from build123d import *

# Parameters (mm, degrees)
BOSS_EXTRUDE1_DEPTH  = 100
BOSS_EXTRUDE2_DEPTH  = 10
BOSS_EXTRUDE2_DRAFT  = 45
SKETCH3_R            = 34.5
BOSS_EXTRUDE3_DEPTH  = 10
SKETCH4_R            = 31
BOSS_EXTRUDE4_DEPTH  = 30
SKETCH5_R            = 2.5
SKETCH5_R_2          = 2
BOSS_EXTRUDE5_DEPTH  = 1
CIRPATTERN1_COUNT    = 12
BOSS_EXTRUDE6_DEPTH  = 100
SKETCH7_R            = 31
BOSS_EXTRUDE7_DEPTH  = 10
SKETCH8_R            = 30
BOSS_EXTRUDE8_DEPTH  = 1
SKETCH9_R            = 31
BOSS_EXTRUDE9_DEPTH  = 10
SKETCH11_R           = 42.5
BOSS_EXTRUDE10_DEPTH = 10.5
BOSS_EXTRUDE11_DEPTH = 35
BOSS_EXTRUDE12_DEPTH = 40
CUT_EXTRUDE1_DEPTH   = 40
SKETCH16_R           = 15
CUT_EXTRUDE2_DEPTH   = 20
SKETCH17_R           = 15
CUT_EXTRUDE3_DEPTH   = 20


with BuildPart() as part:
    # Sketch1 → Boss-Extrude1 (new body)
    with BuildSketch(Plane(origin=(0, 0, 0), x_dir=(1, 0, 0), z_dir=(0, 1, 0))):
        with BuildLine():
            Line((-37.5, 45), (37.5, 45))
            ThreePointArc((37.5, 45), (45.880962103, 0), (37.5, -45))
            Line((37.5, -45), (-37.5, -45))
            ThreePointArc((-37.5, -45), (-45.880962103, 0), (-37.5, 45))
        make_face()
    extrude(amount=BOSS_EXTRUDE1_DEPTH)


with BuildPart() as boss_extrude2_tool:
    # Sketch2 → Boss-Extrude2 (with draft: the straight prism first)
    with BuildSketch(Plane(origin=(0, 100, 0), x_dir=(1, 0, 0), z_dir=(0, 1, 0))):
        with BuildLine():
            Line((37.5, 45), (-37.5, 45))
            ThreePointArc((-37.5, 45), (-45.880962103, 0), (-37.5, -45))
            Line((-37.5, -45), (37.5, -45))
            ThreePointArc((37.5, -45), (45.880962103, 0), (37.5, 45))
        make_face()
    extrude(amount=BOSS_EXTRUDE2_DEPTH)
    # Boss-Extrude2: the draft: its side faces are tilted about the plane it starts from
    boss_extrude2_sides = [boss_extrude2_tool.faces().sort_by_distance(p)[0] for p in [
        (0, 105, -45),
        (-45.880962103, 105, 0),
        (0, 105, 45),
        (45.880962103, 105, 0),
    ]]
    draft(boss_extrude2_sides, Plane(origin=(0, 100, 0), x_dir=(1, 0, 0), z_dir=(0, 1, 0)), BOSS_EXTRUDE2_DRAFT)


with BuildPart() as part_1:
    add(part.part)

    # Boss-Extrude2: add boss_extrude2_tool
    add(boss_extrude2_tool.part)

    # Sketch3 → Boss-Extrude3 (add)
    with BuildSketch(Plane(origin=(0, 110, 0), x_dir=(1, 0, 0), z_dir=(0, 1, 0))):
        with Locations(Location((0, 0, 0), (0, 0, 270))):
            Circle(SKETCH3_R)
    extrude(amount=BOSS_EXTRUDE3_DEPTH)

    # Sketch4 → Boss-Extrude4 (add)
    with BuildSketch(Plane(origin=(0, 120, 0), x_dir=(1, 0, 0), z_dir=(0, 1, 0))):
        with Locations(Location((0, 0, 0), (0, 0, 270))):
            Circle(SKETCH4_R)
    extrude(amount=BOSS_EXTRUDE4_DEPTH)

    # Sketch5 → Boss-Extrude5 (add)
    with BuildSketch(Plane(origin=(0, 150, 0), x_dir=(1, 0, 0), z_dir=(0, 1, 0))):
        with Locations(Location((27, 0, 0), (0, 0, 270))):
            Circle(SKETCH5_R)
        with Locations(Location((27, 0, 0), (0, 0, 270))):
            Circle(SKETCH5_R_2, mode=Mode.SUBTRACT)
    boss_extrude5 = extrude(amount=BOSS_EXTRUDE5_DEPTH)

    # CirPattern1: Boss-Extrude5 ×12 about axis
    cirpattern1_axis = Axis((0, 0, 0), (0, 1, 0))
    for i in range(1, CIRPATTERN1_COUNT):
        add(boss_extrude5.rotate(cirpattern1_axis, i * 360 / CIRPATTERN1_COUNT))

    # Sketch6 → Boss-Extrude6 (add)
    with BuildSketch(Plane(origin=(0, 150, 0), x_dir=(1, 0, 0), z_dir=(0, 1, 0))):
        with BuildLine():
            Line((16, 17), (16, -17))
            ThreePointArc((16, -17), (0, -23.900331129), (-16, -17))
            Line((-16, -17), (-16, 17))
            ThreePointArc((-16, 17), (0, 23.900331129), (16, 17))
        make_face()
    extrude(amount=BOSS_EXTRUDE6_DEPTH)

    # Sketch7 → Boss-Extrude7 (add)
    with BuildSketch(Plane(origin=(0, 250, 0), x_dir=(1, 0, 0), z_dir=(0, 1, 0))):
        with Locations(Location((0, 0, 0), (0, 0, 270))):
            Circle(SKETCH7_R)
    extrude(amount=BOSS_EXTRUDE7_DEPTH)

    # Sketch8 → Boss-Extrude8 (add)
    with BuildSketch(Plane(origin=(0, 260, 0), x_dir=(1, 0, 0), z_dir=(0, 1, 0))):
        with Locations(Location((0, 0, 0), (0, 0, 270))):
            Circle(SKETCH8_R)
    extrude(amount=BOSS_EXTRUDE8_DEPTH)

    # Sketch9 → Boss-Extrude9 (add)
    with BuildSketch(Plane(origin=(0, 261, 0), x_dir=(1, 0, 0), z_dir=(0, 1, 0))):
        with Locations(Location((0, 0, 0), (0, 0, 270))):
            Circle(SKETCH9_R)
    extrude(amount=BOSS_EXTRUDE9_DEPTH)

    # Sketch11 → Boss-Extrude10 (add, symmetric)
    with BuildSketch(Plane.ZY.offset(-37.5)):
        Circle(SKETCH11_R)
    extrude(amount=BOSS_EXTRUDE10_DEPTH, both=True)

    # Sketch12 → Boss-Extrude11 (add)
    with BuildSketch(Plane.ZY.offset(-27)):
        with BuildLine():
            Line((-20, 0), (20, 0))
            Line((20, 0), (20, -30))
            ThreePointArc((20, -30), (0, -37.639320225), (-20, -30))
            Line((-20, -30), (-20, 0))
        make_face()
    extrude(amount=BOSS_EXTRUDE11_DEPTH)

    # Sketch14 → Boss-Extrude12 (add)
    with BuildSketch(Plane(origin=(0, 0, -20), x_dir=(-1, 0, 0), z_dir=(0, 0, -1))):
        with BuildLine():
            Line((8, 0), (8, -42))
            ThreePointArc((8, -42), (25.421855105, -23.929675658), (33, 0))
            Line((33, 0), (8, 0))
        make_face()
    extrude(amount=-BOSS_EXTRUDE12_DEPTH)

    # Sketch15 → Cut-Extrude1 (cut)
    with BuildSketch(Plane(origin=(-8, 0, 0), x_dir=(0, 0, -1), z_dir=(1, 0, 0))):
        with BuildLine():
            Line((-20, -30), (-20, -42))
            Line((-20, -42), (20, -42))
            Line((20, -42), (20, -30))
            ThreePointArc((20, -30), (0, -37.639320225), (-20, -30))
        make_face()
    extrude(amount=-CUT_EXTRUDE1_DEPTH, mode=Mode.SUBTRACT)

    # Sketch16 → Cut-Extrude2 (cut)
    with BuildSketch(Plane(origin=(0, 271, 0), x_dir=(1, 0, 0), z_dir=(0, 1, 0))):
        with Locations(Location((0, 0, 0), (0, 0, 270))):
            Circle(SKETCH16_R)
    extrude(amount=-CUT_EXTRUDE2_DEPTH, mode=Mode.SUBTRACT)

    # Sketch17 → Cut-Extrude3 (cut)
    with BuildSketch(Plane(origin=(48, 0, 0), x_dir=(0, 0, -1), z_dir=(1, 0, 0))):
        Circle(SKETCH17_R)
    extrude(amount=-CUT_EXTRUDE3_DEPTH, mode=Mode.SUBTRACT)


solid = part_1.part
For this review, take the finished solid that the model builds, in its own axes (mm). A direction names the side the tool comes from. Give positions to 0.01 mm unless a question says otherwise; leave off trailing zeros. Loops run counter-clockwise (first coordinate to the right, second up) from the corner with the lowest first, then second, coordinate; pieces in that order, holes last. Notation, with made-up numbers: M -33,24 L 23,24 A24 cw 23,58 Z; hole C -23,50.25 d8. An arc over 180 degrees is marked long. Answer as a JSON object with one key per item and string values. Group by question number.
Q1. Add section C-C on y = 67. Give the boundary of the cut face in (x, z).
Q2. Insertion check: P1, Ø2.5, axis at x = 27, z = 0, coming from the -Y side; P2, Ø9, axis at x = -5.5, y = -19, coming from the -Z side; P3, Ø1, axis at y = 67, z = 31, coming from the +X side. Each pin has a flat end and moves straight along its axis. Give the tip position at first contact, or say it passes through.
Q3. Add section B-B on y = 207.5. Give the boundary of the cut face in (x, z), and give its area (3 significant figures).
Q4. Tool access review of faces 4 (the cylindrical face through (39.69, -41.49, -9.21)), 5 (the flat face through (-32.1, 110, -13.1)), 6 (the flat face through (28, 260, -12)): name each direction out of +Z, -Z, +X, -X, +Y, -Y from which nothing blocks a thin tool from reaching the whole face with its end or side.
Q5. Add section D-D on y = -12. Give the boundary of the cut face in (x, z), and give its area (3 significant figures).
Q6. Add section A-A on y = 139.5. Give the boundary of the cut face in (x, z), and give its area (3 significant figures).
Q7. For probe 1 along X at (y, z) = (264.5, 0); probe 2 along Y at (x, z) = (-19, 30); probe 3 along Y at (x, z) = (-12.5, -31), list the stretches that pass through material, from the lowest coordinate up. Write a range as [from, to].
Q8. Mouldability with a two-part tool opening along Z and no side actions: class faces 1 (the flat face through (27, -35, -13)), 2 (the cylindrical face through (38.14, 0.66, 14.985)), 3 (the cylindrical face through (45.88, 60.41, -0.64)) as +Z half, -Z half, draft (parallel to the pull), parting line (faces both ways), or undercut.
Checked values:
{
 "1": {"outline": "M -37.5,-45 L 37.5,-45 A125 ccw 37.5,45 L -37.5,45 A125 ccw Z"},
 "2": {"P1": "y = -42.5", "P2": "z = -20", "P3": "x = 42.1"},
 "3": {"outline": "M -16,-17 A22 ccw 16,-17 L 16,17 A22 ccw -16,17 Z", "area": "1,390 mm²"},
 "4": {"face 4": "+X", "face 5": "+Y", "face 6": "none"},
 "5": {"outline": "M -30.72,-20 L 27,-20 L 27,-40.77 L 48,-40.77 L 48,-9 L 28,-9 L 28,9 L 48,9 L 48,40.77 L 27,40.77 L 27,20 L -30.72,20 Z", "area": "3,660 mm²"},
 "6": {"outline": "C 0,0 d62", "area": "3,020 mm²"},
 "7": {"probe 1": "[-31, -15], [15, 31]", "probe 2": "[0, 110]", "probe 3": "[0, 120]"},
 "8": {"face 1": "draft", "face 2": "undercut", "face 3": "parting line"}
}
